```python
from build123d import *

# Parameters (mm, degrees)
SKETCH1_R           = 45
SKETCH1_R_2         = 12.5
BOSS_EXTRUDE1_DEPTH = 3.175
SKETCH3_R           = 5
CUT_EXTRUDE1_DEPTH  = 6.35
SKETCH4_R           = 1.25
CUT_EXTRUDE2_DEPTH  = 1


with BuildPart() as part:
    # Sketch1 → Boss-Extrude1 (new body)
    with BuildSketch(Plane(origin=(0, 0, 0), x_dir=(1, 0, 0), z_dir=(0, 1, 0))):
        with Locations(Location((0, 0, 0), (0, 0, 270))):
            Circle(SKETCH1_R)
        with Locations(Location((0, 22.5, 0), (0, 0, 270))):
            Circle(SKETCH1_R_2, mode=Mode.SUBTRACT)
        with Locations(Location((19.485571585, -11.25, 0), (0, 0, 270))):
            Circle(SKETCH1_R_2, mode=Mode.SUBTRACT)
        with Locations(Location((-19.485571585, -11.25, 0), (0, 0, 270))):
            Circle(SKETCH1_R_2, mode=Mode.SUBTRACT)
    extrude(amount=BOSS_EXTRUDE1_DEPTH)

    # Sketch3 → Cut-Extrude1 (cut)
    with BuildSketch(Plane(origin=(0, 3.175, 0), x_dir=(1, 0, 0), z_dir=(0, 1, 0))):
        with Locations(Location((0, 0, 0), (0, 0, 270))):
            Circle(SKETCH3_R)
    extrude(amount=-CUT_EXTRUDE1_DEPTH, mode=Mode.SUBTRACT)

    # Sketch4 → Cut-Extrude2 (cut)
    with BuildSketch(Plane.XZ):
        with Locations(Location((0, 12.5, 0), (0, 0, 270))):
            Circle(SKETCH4_R)
        with Locations(Location((10.825317547, -6.25, 0), (0, 0, 90))):
            Circle(SKETCH4_R)
        with Locations(Location((-10.825317547, -6.25, 0), (0, 0, 90))):
            Circle(SKETCH4_R)
    extrude(amount=-CUT_EXTRUDE2_DEPTH, mode=Mode.SUBTRACT)


solid = part.part
```
Source: CAD feature listing. Evaluate the final solid. Frame: model axes, mm. A direction names the side the tool comes from. Coordinates: 2 decimals unless noted, no trailing zeros. Write each loop counter-clockwise with the first axis right and the second up, starting at its lowest first coordinate (ties: lowest second). Pieces come first, ordered by that corner, then holes. Notation, with made-up numbers: (21.25, -11) -> (28.25, -11) arc R28 cw to (28.25, 21) -> close; hole circle Ø7 at (-32.75, 24). An arc over 180 degrees is marked (long way). Return JSON: item names as keys, results as strings. Group by question number.
1) Section query D-D, the plane y = 2.25. Return loops of the section in (x, z), plus the area to 3 significant figures.
2) Contact query for flat-ended pins moving along their axis: P1, Ø1, axis at y = 3, z = -30, coming from the +X side; P2, Ø0.8, axis at x = -11.5, z = -6, coming from the -Y side; P3, Ø1, axis at x = -6, y = 1, coming from the +Z side. Output: stop coordinate, or through.
3) Section query C-C, the plane x = 27. Return loops of the section in (y, z) (3 decimals), plus the area to 3 significant figures.
4) Section query A-A, the plane x = 0. Return loops of the section in (y, z) (3 decimals).
5) Set-up query: faces 1 (the face through (9.98, 0.49, -7.17)), 2 (the face through (-11.037, 1.565, 2.037)). Return all of +Z, -Z, +X, -X, +Y, -Y with unobstructed straight access to the full face (end or side cutting, diameter ignored); none if empty.
6) Ray query, line 1 along X through (y, z) = (1.85, 11.25); line 2 along X through (y, z) = (2.6, 16); line 3 along X through (y, z) = (0.2, 2). Return the intervals inside material, ascending.
7) Mould query, pull axis Z, two halves, no side actions, for faces 3 (the face through (-17.235, 1.565, 41.569)), 4 (the face through (-12.065, 0.493, -6.413)), 5 (the face through (1, 3.175, 9)). Classes: +Z half, -Z half, draft (parallel to the pull), parting line (faces both ways), or undercut.
8) Section query B-B, the plane z = -22. Return loops of the section in (x, y) (3 decimals), plus the area to 3 significant figures.
From the geometry:
{
 "1": {"outline": "circle Ø90 at (0, 0); hole circle Ø25 at (-19.49, 11.25); hole circle Ø25 at (0, -22.5); hole circle Ø10 at (0, 0); hole circle Ø25 at (19.49, 11.25)", "area": "4,810 mm²"},
 "2": {"P1": "x = 33.98", "P2": "y = 1", "P3": "z = 44.66"},
 "3": {"outline": "(0, -36) -> (3.175, -36) -> (3.175, 1.261) -> (0, 1.261) -> close; (0, 21.239) -> (3.175, 21.239) -> (3.175, 36) -> (0, 36) -> close", "area": "165 mm²"},
 "4": {"outline": "(0, -45) -> (3.175, -45) -> (3.175, -35) -> (0, -35) -> close; (0, -10) -> (3.175, -10) -> (3.175, -5) -> (0, -5) -> close; (0, 5) -> (3.175, 5) -> (3.175, 45) -> (0, 45) -> (0, 13.75) -> (1, 13.75) -> (1, 11.25) -> (0, 11.25) -> close"},
 "5": {"face 1": "-Y", "face 2": "+Y, -Y"},
 "6": {"line 1": "-43.57 to -31.99, -6.99 to 6.99, 31.99 to 43.57", "line 2": "-42.06 to -31.05, -7.92 to 7.92, 31.05 to 42.06", "line 3": "-44.96 to -27.89, -11.08 to -4.58, 4.58 to 11.08, 27.89 to 44.96"},
 "7": {"face 3": "parting line", "face 4": "undercut", "face 5": "draft"},
 "8": {"outline": "(-39.256, 0) -> (-12.49, 0) -> (-12.49, 3.175) -> (-39.256, 3.175) -> close; (12.49, 0) -> (39.256, 0) -> (39.256, 3.175) -> (12.49, 3.175) -> close", "area": "170 mm²"}
}
